```python
from build123d import *

# Parameters (mm, degrees)
F0_W     = 68.180988
F0_H     = 84.445938
F0_W_2   = 29.534492
F0_H_2   = 45.799442
F1_DEPTH = 2


with BuildPart() as f1:
    # F0 (on Top) → F1 (new body)
    with BuildSketch(Plane.XY):
        Rectangle(F0_W, F0_H)
        Polygon((-33.590494, 40.736501), (-33.590494, 41.722969), (-32.604026, 41.722969), (32.604026, 41.722969), (33.590494, 41.722969), (33.590494, 40.736501), (33.590494, -40.736501), (33.590494, -41.722969), (32.604026, -41.722969), (-32.604026, -41.722969), (-33.590494, -41.722969), (-33.590494, -40.736501), align=None, mode=Mode.SUBTRACT)
        Polygon((-15.267246, -22.413252), (-33.590494, -40.736501), (-33.590494, -41.722969), (-32.604026, -41.722969), (-14.280777, -23.399721), (-15.267246, -23.399721), align=None)
        Polygon((-32.604026, 41.722969), (-33.590494, 41.722969), (-33.590494, 40.736501), (-15.267246, 22.413252), (-15.267246, 23.399721), (-14.280777, 23.399721), align=None)
        Polygon((33.590494, 41.722969), (32.604026, 41.722969), (14.280777, 23.399721), (15.267246, 23.399721), (15.267246, 22.413252), (33.590494, 40.736501), align=None)
        Polygon((14.280777, -23.399721), (32.604026, -41.722969), (33.590494, -41.722969), (33.590494, -40.736501), (15.267246, -22.413252), (15.267246, -23.399721), align=None)
        Polygon((-15.267246, 23.399721), (-15.267246, 22.413252), (-15.267246, -22.413252), (-15.267246, -23.399721), (-14.280777, -23.399721), (14.280777, -23.399721), (15.267246, -23.399721), (15.267246, -22.413252), (15.267246, 22.413252), (15.267246, 23.399721), (14.280777, 23.399721), (-14.280777, 23.399721), align=None)
        Rectangle(F0_W_2, F0_H_2, mode=Mode.SUBTRACT)
    extrude(amount=F1_DEPTH)


solid = f1.part
```
The listing builds one solid part. Answer for the finished solid, in the listing's coordinates (mm). A direction names the side the tool comes from. Coordinates: 2 decimals unless noted, no trailing zeros. Loops run counter-clockwise (first coordinate to the right, second up) from the corner with the lowest first, then second, coordinate; pieces in that order, holes last. Notation, with made-up numbers: (48.25, 37) - (104.25, 37) arc R12 cw to (104.25, 59) - close; hole circle Ø10 at (75, 63.5). An arc over 180 degrees is marked (long way). Write item = value, one per line.
1) Find the intervals of material crossed by line 1 along X through (y, z) = (-4, 1.2); line 2 along Y through (x, z) = (0, 1.2); line 3 along X through (y, z) = (-37, 0.6), in increasing order.
Responses:
line_1 = -34.09 to -33.59, -15.27 to -14.77, 14.77 to 15.27, 33.59 to 34.09
line_2 = -42.22 to -41.72, -23.4 to -22.9, 22.9 to 23.4, 41.72 to 42.22
line_3 = -34.09 to -33.59, -29.85 to -27.88, 27.88 to 29.85, 33.59 to 34.09
2) Section C-C (z = 0.85) is taken. Determine the outline of the cut face in (x, y).
Responses:
outline = (-34.09, -42.22) - (34.09, -42.22) - (34.09, 42.22) - (-34.09, 42.22) - close; hole (-33.59, -40.74) - (-15.27, -22.41) - (-15.27, 22.41) - (-33.59, 40.74) - close; hole (-32.6, -41.72) - (32.6, -41.72) - (14.28, -23.4) - (-14.28, -23.4) - close; hole (-32.6, 41.72) - (-14.28, 23.4) - (14.28, 23.4) - (32.6, 41.72) - close; hole (-14.77, -22.9) - (14.77, -22.9) - (14.77, 22.9) - (-14.77, 22.9) - close; hole (15.27, -22.41) - (33.59, -40.74) - (33.59, 40.74) - (15.27, 22.41) - close
3) Section B-B (x = -12) is taken. Determine the outline of the cut face in (y, z).
Responses:
outline = (-42.22, 0) - (-41.72, 0) - (-41.72, 2) - (-42.22, 2) - close; (-23.4, 0) - (-22.9, 0) - (-22.9, 2) - (-23.4, 2) - close; (22.9, 0) - (23.4, 0) - (23.4, 2) - (22.9, 2) - close; (41.72, 0) - (42.22, 0) - (42.22, 2) - (41.72, 2) - close
4) Determine the mould class of faces 3 (the face through (0, 41.723, 1)), 4 (the face through (15, 0, 0)), 5 (the face through (34.09, -1, 1)) for opening direction X: pulls with the +X half, pulls with the -X half, needs draft (parallel to the pull), parting line crosses it, or undercut.
Responses:
face_3 = undercut
face_4 = needs draft
face_5 = pulls with the +X half
5) Section A-A (y = -8.5) is taken. Determine the outline of the cut face in (x, z).
Responses:
outline = (-34.09, 0) - (-33.59, 0) - (-33.59, 2) - (-34.09, 2) - close; (-15.27, 0) - (-14.77, 0) - (-14.77, 2) - (-15.27, 2) - close; (14.77, 0) - (15.27, 0) - (15.27, 2) - (14.77, 2) - close; (33.59, 0) - (34.09, 0) - (34.09, 2) - (33.59, 2) - close
6) Which of the six approach directions +Z, -Z, +X, -X, +Y, -Y give full straight-line access (tool end or side, diameter ignored) to faces 1 (the face through (-24.557, 31.703, 0.986)), 2 (the face through (-34.09, -1, 1))?
Responses:
face_1 = +Z, -Z
face_2 = +Z, -Z, -X, +Y, -Y
